```python
from build123d import *

# Parameters (mm, degrees)
F0_R     = 9.525
F0_R_2   = 5
F1_DEPTH = 7
F2_R     = 5
F3_DEPTH = 48
F4_R     = 5
F5_DEPTH = 12.5


with BuildPart() as f1:
    # F0 (on Top) → F1 (new body, symmetric)
    with BuildSketch(Plane.XY):
        Circle(F0_R)
        Circle(F0_R_2, mode=Mode.SUBTRACT)
    extrude(amount=F1_DEPTH, both=True)

    # F2 (on Front) → F3 (join)
    with BuildSketch(Plane.XZ):
        Circle(F2_R)
    extrude(amount=F3_DEPTH)

    # F4 (on Top) → F5 (cut, symmetric)
    with BuildSketch(Plane.XY):
        Circle(F4_R)
    extrude(amount=F5_DEPTH, both=True, mode=Mode.SUBTRACT)


solid = f1.part
```
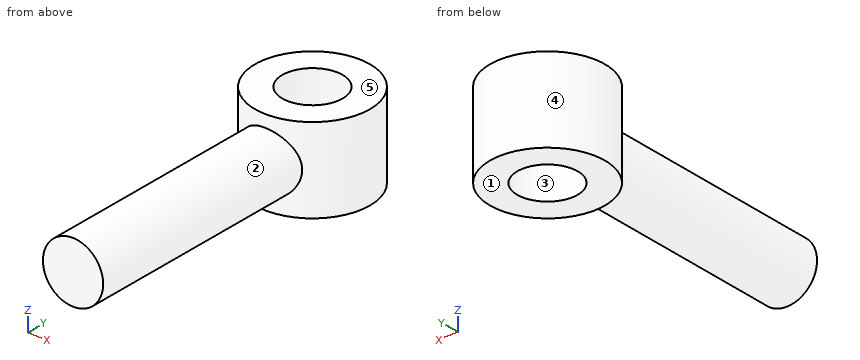
Work out the finished part from the listing and answer in its coordinate system (mm). Face numbers are marked on the shaded views. A direction names the side the tool comes from. Round coordinates to 2 decimals unless told otherwise and drop trailing zeros. Write each loop counter-clockwise with the first axis right and the second up, starting at its lowest first coordinate (ties: lowest second). Pieces come first, ordered by that corner, then holes.
1) A cutting plane is placed at D-D on x = -3.5. Determine the outline of the cut face in (y, z), and give its area (3 significant figures).
2) A cutting plane is placed at B-B on y = 0. Determine the outline of the cut face in (x, z) (3 decimals), and give its area (3 significant figures).
3) Which of the six approach directions +Z, -Z, +X, -X, +Y, -Y give full straight-line access (tool end or side, diameter ignored) to the marked faces 1 and 2?
4) Determine the mould class of the marked faces 3, 4 and 5 for opening direction Y: pulls with the +Y half, pulls with the -Y half, needs draft (parallel to the pull), parting line crosses it, or undercut.
5) A cutting plane is placed at C-C on z = 0. Determine the outline of the cut face in (x, y) (3 decimals), and give its area (3 significant figures).
6) Consider probe 1 along Y at (x, z) = (0, -3.25) (3 decimals); probe 2 along Y at (x, z) = (4.5, -2); probe 3 along X at (y, z) = (2.5, 1.5). Determine where each line is inside the solid, lowest interval first.
7) A cutting plane is placed at A-A on x = 0. Determine the outline of the cut face in (y, z) (3 decimals), and give its area (3 significant figures).
8) Flat-ended cylindrical pins translate along their axes: P1, Ø6, axis at y = -7, z = 0, coming from the -X side; P2, Ø1.5, axis at y = -18.5, z = 5, coming from the -X side; P3, Ø1.5, axis at y = -31, z = 2, coming from the +X side. Find the tip coordinate at first contact, or state that the pin passes through.
Entries:
1. outline: (-48, -3.57) - (-8.86, -3.57) - (-8.86, -7) - (-3.57, -7) - (-3.57, 7) - (-8.86, 7) - (-8.86, 3.57) - (-48, 3.57) - close; (3.57, -7) - (8.86, -7) - (8.86, 7) - (3.57, 7) - close
1. area: 428 mm2
2. outline: (-9.525, -7) - (-5, -7) - (-5, 7) - (-9.525, 7) - close; (5, -7) - (9.525, -7) - (9.525, 7) - (5, 7) - close
2. area: 127 mm2
3. face 1: -Z, +X, -X, +Y, -Y
3. face 2: -Y
4. face 3: undercut
4. face 4: parting line crosses it
4. face 5: needs draft
5. outline: (-5, -48) - (5, -48) - (5, -8.107) arc R9.525 ccw (long way) to (-5, -8.107) - close; hole circle Ø10 at (0, 0)
5. area: 596 mm2
6. probe 1: y = -48 to -5, 5 to 9.525
6. probe 2: y = -48 to -2.18, 2.18 to 8.39
6. probe 3: x = -9.19 to -4.33, 4.33 to 9.19
7. outline: (-48, -5) - (-9.525, -5) - (-9.525, -7) - (-5, -7) - (-5, 7) - (-9.525, 7) - (-9.525, 5) - (-48, 5) - close; (5, -7) - (9.525, -7) - (9.525, 7) - (5, 7) - close
7. area: 511 mm2
8. P1: stops at x = -8.64
8. P2: stops at x = -2.63
8. P3: stops at x = 4.84
